Check sheet for the modelled part. Datum: model origin and axes. Units: mm. Face numbers are marked on the shaded views. Give positions to 0.01 mm unless a question says otherwise; leave off trailing zeros. Loops run counter-clockwise (first coordinate to the right, second up) from the corner with the lowest first, then second, coordinate; pieces in that order, holes last. Notation, with made-up numbers: (62, 31.25) -> (99, 31.25) arc R19 ccw to (99, 36.25) -> close; hole circle Ø10 at (0.25, 20). An arc over 180 degrees is marked (long way). Write each question's results on one line, items separated by ' | '. Start each with the question number.
1. Mould release check, pull along Y, two halves, no side actions. Record for the marked faces 1 and 2: +Y half, -Y half, draft (parallel to the pull), parting line (faces both ways), or undercut.
2. Cross-section at D-D on x = 0. Record the boundary of the cut face in (y, z), and give its area (3 significant figures).
3. Material ranges on L1, parallel to Y at x = 0, z = 3.6; L2, parallel to X at y = -0.75, z = 7.25; L3, parallel to Z at x = -0.25, y = 8.75, recorded low to high. Write a range as from..to.
4. Gauge pin test, flat ends, axial feed: pin 1 Ø1 at (y, z) = (9, 2) entering from -X; pin 2 Ø0.6 at (x, z) = (3, 6.5) entering from -Y; pin 3 Ø2 at (x, y) = (4.5, -4.5) entering from +Z. Record the tip position at first contact, or that the pin passes through.
5. Cross-section at B-B on z = 7.75. Record the boundary of the cut face in (x, y).
6. Cross-section at C-C on y = 0. Record the boundary of the cut face in (x, z), and give its area (3 significant figures).
7. Cross-section at A-A on z = 4.25. Record the boundary of the cut face in (x, y), and give its area (3 significant figures).
from build123d import *

# Parameters (mm, degrees)
SKETCH1_R           = 12.5
BOSS_EXTRUDE1_DEPTH = 5
SKETCH2_R           = 11.5
CUT_EXTRUDE1_DEPTH  = 2.5
BOSS_EXTRUDE2_DEPTH = 2.6
SKETCH4_W           = 1.2
SKETCH4_H           = 3
BOSS_EXTRUDE3_DEPTH = 4
BOSS_EXTRUDE4_START = 3
SKETCH5_R           = 12.5
BOSS_EXTRUDE4_DEPTH = 3


with BuildPart() as part:
    # Sketch1 → Boss-Extrude1 (new body)
    with BuildSketch(Plane.XY):
        Circle(SKETCH1_R)
    extrude(amount=BOSS_EXTRUDE1_DEPTH)

    # Sketch2 → Cut-Extrude1 (cut)
    with BuildSketch(Plane.XY.offset(5)):
        Circle(SKETCH2_R)
    extrude(amount=-CUT_EXTRUDE1_DEPTH, mode=Mode.SUBTRACT)

    # Sketch3 → Boss-Extrude2 (add)
    with BuildSketch(Plane.XY.offset(2.5)):
        Polygon((-2.2665, 0.415113025), (2.2665, 0.415113025), (2.2665, 1.506034439), (3.4665, 1.506034439), (3.4665, -1.493965561), (2.2665, -1.493965561), (2.2665, -0.403044147), (-2.2665, -0.403044147), (-2.2665, -1.493965561), (-3.4665, -1.493965561), (-3.4665, 1.506034439), (-2.2665, 1.506034439), align=None)
    extrude(amount=BOSS_EXTRUDE2_DEPTH)

    # Sketch4 → Boss-Extrude3 (add)
    with BuildSketch(Plane.XY.offset(5.1)):
        with Locations((-2.8665, 0.006034439)):
            Rectangle(SKETCH4_W, SKETCH4_H)
        with Locations((2.8665, 0.006034439)):
            Rectangle(SKETCH4_W, SKETCH4_H)
    extrude(amount=BOSS_EXTRUDE3_DEPTH)

    # Sketch5 → Boss-Extrude4 (add)
    with BuildSketch(Plane(origin=(0, 0, 0), x_dir=(-1, 0, 0), z_dir=(0, 0, -1)).offset(BOSS_EXTRUDE4_START)):
        Circle(SKETCH5_R)
    extrude(amount=-BOSS_EXTRUDE4_DEPTH)


solid = part.part
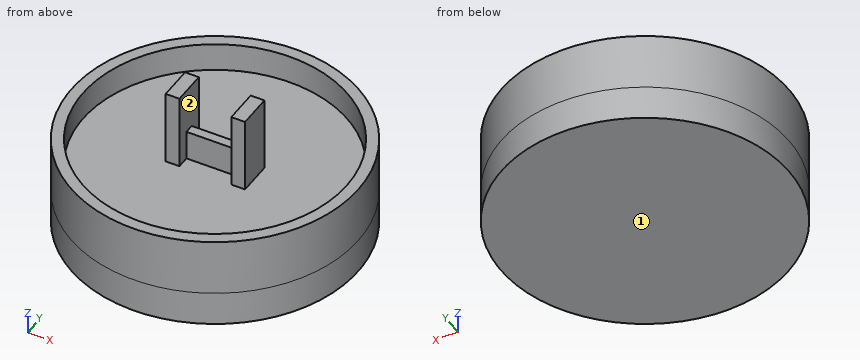
Geometry says:
1) face 1: draft | face 2: undercut
2) outline: (-12.5, -3) -> (12.5, -3) -> (12.5, 5) -> (11.5, 5) -> (11.5, 2.5) -> (0.42, 2.5) -> (0.42, 5.1) -> (-0.4, 5.1) -> (-0.4, 2.5) -> (-11.5, 2.5) -> (-11.5, 5) -> (-12.5, 5) -> close | area: 145 mm^2
3) L1: -12.5..-11.5, -0.4..0.42, 11.5..12.5 | L2: -3.47..-2.27, 2.27..3.47 | L3: -3..2.5
4) pin 1: x = -9.17 | pin 2: y = -1.49 | pin 3: z = 2.5
5) outline: (-3.47, -1.49) -> (-2.27, -1.49) -> (-2.27, 1.51) -> (-3.47, 1.51) -> close; (2.27, -1.49) -> (3.47, -1.49) -> (3.47, 1.51) -> (2.27, 1.51) -> close
6) outline: (-12.5, -3) -> (12.5, -3) -> (12.5, 5) -> (11.5, 5) -> (11.5, 2.5) -> (3.47, 2.5) -> (3.47, 9.1) -> (2.27, 9.1) -> (2.27, 5.1) -> (-2.27, 5.1) -> (-2.27, 9.1) -> (-3.47, 9.1) -> (-3.47, 2.5) -> (-11.5, 2.5) -> (-11.5, 5) -> (-12.5, 5) -> close | area: 170 mm^2
7) outline: circle Ø25 at (0, 0); (-3.47, -1.49) -> (-2.27, -1.49) -> (-2.27, -0.4) -> (2.27, -0.4) -> (2.27, -1.49) -> (3.47, -1.49) -> (3.47, 1.51) -> (2.27, 1.51) -> (2.27, 0.42) -> (-2.27, 0.42) -> (-2.27, 1.51) -> (-3.47, 1.51) -> close; hole circle Ø23 at (0, 0) | area: 86.3 mm^2
